from build123d import *

# Parameters (mm, degrees)
F0_R      = 34.671
F0_R_2    = 9.525
F1_DEPTH  = 12.7
F2_R      = 39.6875
F2_R_2    = 34.671
F3_DEPTH  = 3.175
F1_FACE_R = 9.525
F4_DEPTH  = 3.175


with BuildPart() as f1:
    # F0 (on Right) → F1 (new body)
    with BuildSketch(Plane.YZ):
        Circle(F0_R)
        Circle(F0_R_2, mode=Mode.SUBTRACT)
    extrude(amount=F1_DEPTH)

    # F2 (on face) → F3 (join)
    with BuildSketch(Plane(origin=(0, 0, 0), x_dir=(0, -1, 0), z_dir=(-1, 0, 0))):
        Circle(F2_R)
        Circle(F2_R_2, mode=Mode.SUBTRACT)
    extrude(amount=F3_DEPTH)

    # F1_face (on face) → F4 (join)
    with BuildSketch(Plane(origin=(0, 0, 0), x_dir=(0, 1, 0), z_dir=(-1, 0, 0))):
        with BuildLine():
            ThreePointArc((-34.671, 0), (0, -34.671), (34.671, 0))
            ThreePointArc((34.671, 0), (0, 34.671), (-34.671, 0))
        make_face()
        Circle(F1_FACE_R, mode=Mode.SUBTRACT)
    extrude(amount=F4_DEPTH)


solid = f1.part
Here's how the part is built. I have some questions about the finished solid (model axes, mm). A direction names the side the tool comes from. Round coordinates to 2 decimals unless told otherwise and drop trailing zeros. Order: outer loops, then holes, each group sorted by start corner. A loop starts at its lowest first (then second) coordinate and runs counter-clockwise, first axis right, second up. Notation, with made-up numbers: (37, 25) -> (74, 25) arc R6 cw to (74, 29) -> close; hole circle Ø4 at (45.5, -39). An arc over 180 degrees is marked (long way). Return JSON: item names as keys, results as strings.
Q1. If we mould it in two halves opening along Z, with no side actions, what happens to faces 3 (the cylindrical face through (4.874, -7.559, 5.796)), 4 (the cylindrical face through (6.261, -34.637, 1.524)), 5 (the flat face through (-3.175, 8, 8))? For each: released by +Z, released by -Z, zero draft, split by the parting line, or undercut.
Filled sheet:
{"face 3": "undercut", "face 4": "split by the parting line", "face 5": "zero draft"}
Q2. If we section it at C-C on x = 7: List the corners of the cut face in (y, z) for me (3 decimals), plus the area to 3 significant figures.
Filled sheet:
{"outline": "circle Ø69.342 at (0, 0); hole circle Ø19.05 at (0, 0)", "area": "3,490 mm^2"}
Q3. If we section it at D-D on y = 30.5: List the corners of the cut face in (x, z) for me (3 decimals).
Filled sheet:
{"outline": "(-3.175, -25.394) -> (0, -25.394) -> (0, -16.487) -> (12.7, -16.487) -> (12.7, 16.487) -> (0, 16.487) -> (0, 25.394) -> (-3.175, 25.394) -> close"}
Q4. I need wall thicknesses on line 1 along Z through (x, y) = (7, 0) (3 decimals); line 2 along X through (y, z) = (-16, -33) (3 decimals); line 3 along Z through (x, y) = (5.25, 8). Which ranges of each line are inside material? Lowest first, please. Write a range as from..to.
Filled sheet:
{"line 1": "z = -34.671..-9.525, 9.525..34.671", "line 2": "x = -3.175..0", "line 3": "z = -33.74..-5.17, 5.17..33.74"}
Q5. If we section it at B-B on y = 1: List the corners of the cut face in (x, z) for me (3 decimals).
Filled sheet:
{"outline": "(-3.175, -39.675) -> (0, -39.675) -> (0, -34.657) -> (12.7, -34.657) -> (12.7, -9.472) -> (-3.175, -9.472) -> close; (-3.175, 9.472) -> (12.7, 9.472) -> (12.7, 34.657) -> (0, 34.657) -> (0, 39.675) -> (-3.175, 39.675) -> close"}
Q6. Which directions (+Z, -Z, +X, -X, +Y, -Y) give clear straight access to the entire face, cutting with the end or side of a thin tool? Please do faces 1 (the flat face through (12.7, 7, -7)), 2 (the flat face through (0, 0, -35)).
Filled sheet:
{"face 1": "+Z, -Z, +X, +Y, -Y", "face 2": "+X"}
Q7. If we section it at A-A on z = 0: List the corners of the cut face in (x, y) for me (1 decimal).
Filled sheet:
{"outline": "(-3.2, -39.7) -> (0, -39.7) -> (0, -34.7) -> (12.7, -34.7) -> (12.7, -9.5) -> (-3.2, -9.5) -> close; (-3.2, 9.5) -> (12.7, 9.5) -> (12.7, 34.7) -> (0, 34.7) -> (0, 39.7) -> (-3.2, 39.7) -> close"}
Q8. For pin 1 Ø1 at (x, y) = (11, -23) entering from +Z; pin 2 Ø5 at (x, z) = (10, 18) entering from +Y; pin 3 Ø3 at (x, z) = (0, 21.5) entering from -Y, each with a flat end and sliding along its axis, tell me the tip position at first contact or that it passes through.
Filled sheet:
{"pin 1": "stops at z = 26.38", "pin 2": "stops at y = 31.01", "pin 3": "stops at y = -34.28"}
